```python
from build123d import *

# Parameters (mm, degrees)
OBR_T1_ANGLE                = 90
OBR_T2_ANGLE                = 110
DODANIE_WYCI_GNI_CIE1_DEPTH = 15
SZKIC5_R                    = 30
DODANIE_WYCI_GNI_CIE2_DEPTH = 5
ZAOKR_GLENIE1_R             = 5
DODANIE_WYCI_GNI_CIE3_START = 5
SZKIC6_R                    = 30
DODANIE_WYCI_GNI_CIE3_DEPTH = 5
ZAOKR_GLENIE2_R             = 5


with BuildPart() as part:
    # Szkic1 → Obrót1 (revolve)
    with BuildSketch(Plane(origin=(0, 0, 0), x_dir=(1, 0, 0), z_dir=(0, 1, 0))):
        with BuildLine():
            Line((-20, -55), (-20, 55))
            Line((-20, 55), (-75, 55))
            ThreePointArc((-75, 55), (-93.005376189, 0), (-75, -55))
            Line((-75, -55), (-20, -55))
        make_face()
    revolve(axis=Axis((-20, 0, 55), (0, 0, -1)), revolution_arc=OBR_T1_ANGLE)

    # Szkic2 → Obrót2 (revolve)
    with BuildSketch(Plane(origin=(-20, 0, 0), x_dir=(0, 0, -1), z_dir=(1, 0, 0))):
        with BuildLine():
            Line((-55, 55), (-55, 40))
            Line((-55, 40), (55, 40))
            Line((55, 40), (55, 55))
            Line((55, 55), (55, 95))
            ThreePointArc((55, 95), (0, 109.772492001), (-55, 95))
            Line((-55, 95), (-55, 55))
        make_face()
    revolve(axis=Axis((-20, 40, 55), (0, 0, 1)), revolution_arc=OBR_T2_ANGLE)

    # Szkic3 → Dodanie-wyciągnięcie1 (add)
    with BuildSketch(Plane(origin=(-20, 0, 0), x_dir=(0, 0, -1), z_dir=(1, 0, 0))):
        Polygon((0, 109.772492001), (-25, 109.772492001), (-25, 99.772492001), (25, 99.772492001), (25, 109.772492001), align=None)
    extrude(amount=-DODANIE_WYCI_GNI_CIE1_DEPTH)

    # Szkic5 → Dodanie-wyciągnięcie2 (add)
    with BuildSketch(Plane.XY.offset(55)):
        with Locations(Location((-32.802857824, -0.227507999, 0), (0, 0, 179.565487562))):
            Circle(SZKIC5_R)
    extrude(amount=DODANIE_WYCI_GNI_CIE2_DEPTH)

    # Zaokrąglenie1
    zaokr_glenie1_edges = [part.edges().sort_by_distance(p)[0] for p in [
        (-2.803720502, -0.455015999, 60),
    ]]
    fillet(zaokr_glenie1_edges, radius=ZAOKR_GLENIE1_R - 0.0001)  # a hair under: the kernel refuses the full size

    # Szkic6 → Dodanie-wyciągnięcie3 (add)
    with BuildSketch(Plane(origin=(0, 0, -55), x_dir=(-1, 0, 0), z_dir=(0, 0, -1)).offset(DODANIE_WYCI_GNI_CIE3_START)):
        with Locations(Location((32.802857824, -0.227507999, 0), (0, 0, 115.262238739))):
            Circle(SZKIC6_R)
    extrude(amount=-DODANIE_WYCI_GNI_CIE3_DEPTH)

    # Zaokrąglenie2
    zaokr_glenie2_edges = [part.edges().sort_by_distance(p)[0] for p in [
        (-45.605715649, -27.358428211, -60),
    ]]
    fillet(zaokr_glenie2_edges, radius=ZAOKR_GLENIE2_R - 0.0001)  # a hair under: the kernel refuses the full size


solid = part.part
```
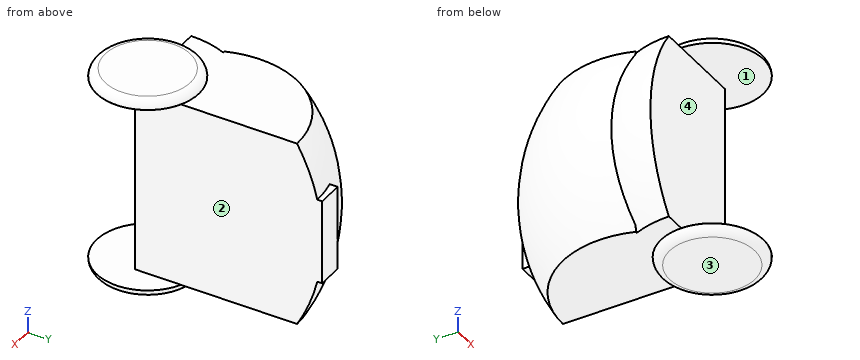
Here's how the part is built. I have some questions about the finished solid (model axes, mm). Face numbers are marked on the shaded views. A direction names the side the tool comes from. Round coordinates to 2 decimals unless told otherwise and drop trailing zeros. One line per question, with ' | ' between items.
1) For pin 1 Ø1.5 at (x, y) = (-29.5, 39) entering from -Z; pin 2 Ø2.5 at (x, y) = (-31, 107.5) entering from -Z; pin 3 Ø8 at (x, z) = (-71, -7.5) entering from -Y, each with a flat end and sliding along its axis, tell me the tip position at first contact or that it passes through.
Working result:
pin 1: z = -55 | pin 2: z = -25 | pin 3: y = 0
2) For the marked faces 1, 2, 3 and 4, which set-ups out of +Z, -Z, +X, -X, +Y, -Y let a thin tool reach every point of the face, with its end or its side?
Working result:
face 1: +X, -Y | face 2: +X, +Y, -Y | face 3: -Z, +X, -X, +Y, -Y | face 4: +X, -X, -Y
3) I need wall thicknesses on line 1 along Z through (x, y) = (-57.5, 72); line 2 along Y through (x, z) = (-33, 14); line 3 along X through (y, z) = (22, -53.5). Which ranges of each line are inside material? Lowest first, please.
Working result:
line 1: -55 to 55 | line 2: 0 to 109.77 | line 3: -72.87 to -20
